Geometry: final body of the model. Coordinates: model frame, mm. Coordinates: 2 decimals unless noted, no trailing zeros. Order: outer loops, then holes, each group sorted by start corner. A loop starts at its lowest first (then second) coordinate and runs counter-clockwise, first axis right, second up. Notation, with made-up numbers: M 42,3 L 60,3 A23 cw 60,39 Z; hole C 11.5,45.5 d9. An arc over 180 degrees is marked long. Write item = value, one per line.
from build123d import *

# Parameters (mm, degrees)
SKETCH1_W               = 90
SKETCH1_H               = 50
BOSS_EXTRUDE1_DEPTH     = 4
CUT_EXTRUDE1_DEPTH      = 104.033974979
CUT_EXTRUDE1_DEPTH_BACK = 104.033974979
SKETCH2_R               = 2.5


with BuildPart() as part:
    # Sketch1 → Boss-Extrude1 (new body)
    with BuildSketch(Plane(origin=(0, 0, 0), x_dir=(0, 0, -1), z_dir=(1, 0, 0))):
        with Locations((45, -25)):
            Rectangle(SKETCH1_W, SKETCH1_H)
    extrude(amount=BOSS_EXTRUDE1_DEPTH)

    # Sketch2 → Cut-Extrude1 (cut, two sides: drawn at the far end of the back side and taken through both)
    with BuildSketch(Plane(origin=(4, 0, 0), x_dir=(0, 0, -1), z_dir=(1, 0, 0)).offset(-CUT_EXTRUDE1_DEPTH_BACK)):
        with Locations((15, -7)):
            Circle(SKETCH2_R)
        with Locations((45, -7)):
            Circle(SKETCH2_R)
        with Locations((75, -7)):
            Circle(SKETCH2_R)
    extrude(amount=CUT_EXTRUDE1_DEPTH + CUT_EXTRUDE1_DEPTH_BACK, mode=Mode.SUBTRACT)


solid = part.part
1) Section B-B, the plane z = -75. Return loops of the section in (x, y).
Numbers:
outline = M 0,-50 L 4,-50 L 4,-9.5 L 0,-9.5 Z; M 0,-4.5 L 4,-4.5 L 4,0 L 0,0 Z
2) Pin query (flat end, axial travel): pin 1 (6 mm diameter, centred on y = -7, z = -75, fed in from -X). Return the tip coordinate at first contact, or that it passes through.
Numbers:
pin_1 = 0
3) Mould query, pull axis Z, two halves, no side actions, for faces 1 (the face through (2, 0, -44)), 2 (the face through (2, -25, 0)), 3 (the face through (2, -6.9, -12.5)). Classes: pulls with the +Z half, pulls with the -Z half, needs draft (parallel to the pull), parting line crosses it, or undercut.
Numbers:
face_1 = needs draft
face_2 = pulls with the +Z half
face_3 = undercut
4) Section A-A, the plane y = -7. Return loops of the section in (x, z).
Numbers:
outline = M 0,-90 L 4,-90 L 4,-77.5 L 0,-77.5 Z; M 0,-72.5 L 4,-72.5 L 4,-47.5 L 0,-47.5 Z; M 0,-42.5 L 4,-42.5 L 4,-17.5 L 0,-17.5 Z; M 0,-12.5 L 4,-12.5 L 4,0 L 0,0 Z
5) Line query: L1, parallel to Z at x = 1.05, y = -7; L2, parallel to Y at x = 1.7, z = -15; L3, parallel to Z at x = 2.75, y = -7.5. Output: solid intervals per line, ascending.
Numbers:
L1 = -90 to -77.5, -72.5 to -47.5, -42.5 to -17.5, -12.5 to 0
L2 = -50 to -9.5, -4.5 to 0
L3 = -90 to -77.45, -72.55 to -47.45, -42.55 to -17.45, -12.55 to 0
